from build123d import *

# Parameters (mm, degrees)
SKETCH5_R               = 2.5
BOSS_EXTRUDE2_DEPTH     = 10
CIRPATTERN2_COUNT       = 2
CUT_EXTRUDE4_REACH      = 84.468
SKETCH7_R               = 1.5
CUT_EXTRUDE5_DEPTH      = 83.46817568
SKETCH10_W              = 7.5
SKETCH10_H              = 20
BOSS_EXTRUDE3_DEPTH     = 50
CUT_EXTRUDE6_REACH      = 113.36
SKETCH11_R              = 3.75
LPATTERN1_COUNT         = 4
LPATTERN1_PITCH         = 10
MIRROR1_COPY_1_REACH    = 113.36
MIRROR1_COPY_1_SKETCH_R = 3.75
MIRROR1_COPY_2_REACH    = 113.36
MIRROR1_COPY_2_SKETCH_R = 3.75
MIRROR1_COPY_3_REACH    = 113.36
MIRROR1_COPY_3_SKETCH_R = 3.75
FILLET1_R               = 2.5


with BuildPart() as part:
    # Sketch4 → Revolve2 (revolve)
    with BuildSketch(Plane(origin=(0, 0, 0), x_dir=(0, 0, -1), z_dir=(1, 0, 0))):
        Polygon((0, 0), (50, 0), (50, -10), (53, -10), (53, 0), (56, 0), (56, 10), (53, 10), (53, 25), (50, 25), (50, 2), (0, 2), align=None)
    revolve(axis=Axis((0, 0, 0), (0, 1, 0)))

    # Sketch5 → Boss-Extrude2 (add)
    with BuildSketch(Plane(origin=(0, 2, 0), x_dir=(1, 0, 0), z_dir=(0, 1, 0))):
        with Locations(Location((-45, 0, 0), (0, 0, 270))):
            Circle(SKETCH5_R)
    boss_extrude2 = extrude(amount=BOSS_EXTRUDE2_DEPTH)

    # CirPattern2: Boss-Extrude2 ×2 about axis
    cirpattern2_axis = Axis((0.112781955, 0, 0), (0, 1, 0))
    for i in range(1, CIRPATTERN2_COUNT):
        add(boss_extrude2.rotate(cirpattern2_axis, i * 360 / CIRPATTERN2_COUNT))

    # Sketch6 → Cut-Extrude4 (cut, up to next)
    with BuildSketch(Plane(origin=(0, 2, 0), x_dir=(1, 0, 0), z_dir=(0, 1, 0)), mode=Mode.PRIVATE) as cut_extrude4_sk1:
        with BuildLine():
            Line((-5.740251485, 13.858192988), (-13.393920133, 32.335783638))
            ThreePointArc((-13.393920133, 32.335783638), (0, 35), (13.393920133, 32.335783638))
            Line((13.393920133, 32.335783638), (5.740251485, 13.858192988))
            ThreePointArc((5.740251485, 13.858192988), (0, 15), (-5.740251485, 13.858192988))
        make_face()
    cut_extrude4_tool1 = extrude(cut_extrude4_sk1.sketch, amount=-CUT_EXTRUDE4_REACH, mode=Mode.PRIVATE) & part.part
    add(cut_extrude4_tool1.solids().sort_by_distance((0, 2, -25.661711))[0], mode=Mode.SUBTRACT)

    # Sketch7 → Cut-Extrude5 (cut, through all)
    with BuildSketch(Plane(origin=(0, 2, 0), x_dir=(1, 0, 0), z_dir=(0, 1, 0))):
        with Locations(Location((0, 0, 0), (0, 0, 270))):
            Circle(SKETCH7_R)
    extrude(amount=-CUT_EXTRUDE5_DEPTH, mode=Mode.SUBTRACT)

    # Sketch10 → Boss-Extrude3 (add)
    with BuildSketch(Plane.XZ):
        with Locations((30, 0)):
            Rectangle(SKETCH10_W, SKETCH10_H)
    boss_extrude3 = extrude(amount=BOSS_EXTRUDE3_DEPTH)

    # Sketch11 → Cut-Extrude6 (cut, up to next)
    with BuildSketch(Plane.ZY.offset(-26.25), mode=Mode.PRIVATE) as cut_extrude6_sk1:
        with Locations((0, -10)):
            Circle(SKETCH11_R)
    cut_extrude6_tool1 = extrude(cut_extrude6_sk1.sketch, amount=-CUT_EXTRUDE6_REACH, mode=Mode.PRIVATE) & part.part
    cut_extrude6 = cut_extrude6_tool1.solids().sort_by_distance((26.25, -10, 0))[0]
    add(cut_extrude6, mode=Mode.SUBTRACT)

    # LPattern1: Cut-Extrude6 ×4
    with Locations(*[(0, -i * LPATTERN1_PITCH, 0) for i in range(1, LPATTERN1_COUNT)]):
        add(cut_extrude6, mode=Mode.SUBTRACT)

    # Mirror1: Boss-Extrude3, Cut-Extrude6 across plane
    add(boss_extrude3.mirror(Plane(origin=(0, 0, 0), x_dir=(0, 0, 1), z_dir=(1, 0, 0))))
    add(cut_extrude6.mirror(Plane(origin=(0, 0, 0), x_dir=(0, 0, 1), z_dir=(1, 0, 0))), mode=Mode.SUBTRACT)

    # Mirror1 copy 1 sketch → Mirror1 copy 1 (cut, up to next)
    with BuildSketch(Plane(origin=(-26.25, -10, 0), x_dir=(0, 0, 1), z_dir=(1, 0, 0)), mode=Mode.PRIVATE) as mirror1_copy_1_sk1:
        with Locations((0, 10)):
            Circle(MIRROR1_COPY_1_SKETCH_R)
    mirror1_copy_1_tool1 = extrude(mirror1_copy_1_sk1.sketch, amount=-MIRROR1_COPY_1_REACH, mode=Mode.PRIVATE) & part.part
    add(mirror1_copy_1_tool1.solids().sort_by_distance((-26.25, -20, 0))[0], mode=Mode.SUBTRACT)

    # Mirror1 copy 2 sketch → Mirror1 copy 2 (cut, up to next)
    with BuildSketch(Plane(origin=(-26.25, -20, 0), x_dir=(0, 0, 1), z_dir=(1, 0, 0)), mode=Mode.PRIVATE) as mirror1_copy_2_sk1:
        with Locations((0, 10)):
            Circle(MIRROR1_COPY_2_SKETCH_R)
    mirror1_copy_2_tool1 = extrude(mirror1_copy_2_sk1.sketch, amount=-MIRROR1_COPY_2_REACH, mode=Mode.PRIVATE) & part.part
    add(mirror1_copy_2_tool1.solids().sort_by_distance((-26.25, -30, 0))[0], mode=Mode.SUBTRACT)

    # Mirror1 copy 3 sketch → Mirror1 copy 3 (cut, up to next)
    with BuildSketch(Plane(origin=(-26.25, -30, 0), x_dir=(0, 0, 1), z_dir=(1, 0, 0)), mode=Mode.PRIVATE) as mirror1_copy_3_sk1:
        with Locations((0, 10)):
            Circle(MIRROR1_COPY_3_SKETCH_R)
    mirror1_copy_3_tool1 = extrude(mirror1_copy_3_sk1.sketch, amount=-MIRROR1_COPY_3_REACH, mode=Mode.PRIVATE) & part.part
    add(mirror1_copy_3_tool1.solids().sort_by_distance((-26.25, -40, 0))[0], mode=Mode.SUBTRACT)

    # Fillet1
    fillet1_edges = [part.edges().sort_by_distance(p)[0] for p in [
        (30, 0, -10),
        (26.25, 0, 0),
        (30, 0, 10),
        (33.75, 0, 0),
        (-30, 0, 10),
        (-33.75, 0, 0),
        (-30, 0, -10),
        (-26.25, 0, 0),
    ]]
    fillet(fillet1_edges, radius=FILLET1_R)


solid = part.part
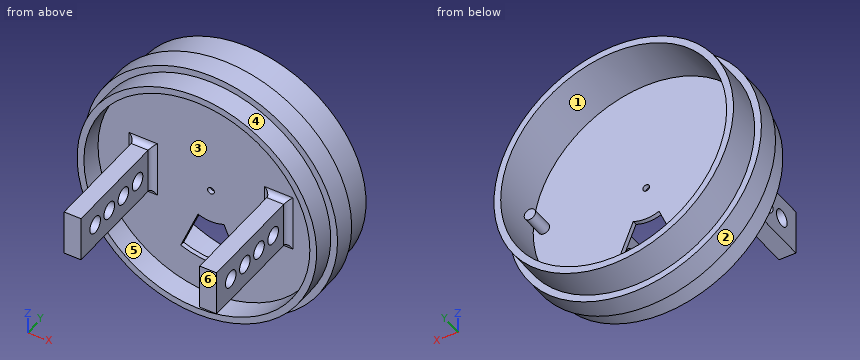
Read the model definition and answer for the solid it produces. Units are mm, in the model's axes. Face numbers are marked on the shaded views. A direction names the side the tool comes from. Round coordinates to 2 decimals unless told otherwise and drop trailing zeros. Write each loop counter-clockwise with the first axis right and the second up, starting at its lowest first coordinate (ties: lowest second). Pieces come first, ordered by that corner, then holes.
1. The part is cut by section C-C, the plane z = 0. State how many separate pieces and enclosed holes the cut face has, then the cut area to 3 significant figures.
2. The part is cut by section D-D, the plane x = -45. Determine the outline of the cut face in (y, z), then the cut area to 3 significant figures.
3. Straight lines are drawn through the part: L1, parallel to Y at x = 28, z = 0; L2, parallel to X at y = 1.4, z = 0; L3, parallel to X at y = 13, z = 0. For each, find the intervals that lie inside material, in ascending order.
4. Which of the six approach directions +Z, -Z, +X, -X, +Y, -Y give full straight-line access (tool end or side, diameter ignored) to the marked faces 1, 2 and 3?
5. The part is cut by section A-A, the plane y = -40. Determine the outline of the cut face in (x, z).
6. The part is cut by section B-B, the plane x = 0. Determine the outline of the cut face in (y, z).
7. Given pin 1 Ø4 at (x, y) = (29, -29) entering from -Z; pin 2 Ø8.5 at (y, z) = (-10, 0) entering from -X; pin 3 Ø12 at (y, z) = (-40, 0) entering from -X, each flat-ended and moving along its own axis, determine where each tip first touches the part or whether it passes through.
8. Determine the mould class of the marked faces 4, 5 and 6 for opening direction X: pulls with the +X half, pulls with the -X half, needs draft (parallel to the pull), parting line crosses it, or undercut.
Values:
1. separate pieces: 10
1. enclosed holes: 0
1. area: 869 mm2
2. outline: (-10, -28) - (0, -28) - (0, -33.33) - (10, -33.33) - (10, -28) - (25, -28) - (25, -21.79) - (2, -21.79) - (2, -2.5) - (12, -2.5) - (12, 2.5) - (2, 2.5) - (2, 21.79) - (25, 21.79) - (25, 28) - (10, 28) - (10, 33.33) - (0, 33.33) - (0, 28) - (-10, 28) - (-10, 21.79) - (0, 21.79) - (0, -21.79) - (-10, -21.79) - close
2. area: 678 mm2
3. L1: y = -50 to -43.75, -36.25 to -33.75, -26.25 to -23.75, -16.25 to -13.75, -6.25 to 2
3. L2: x = -56 to -1.5, 1.5 to 56
3. L3: x = -53 to -50, 50 to 53
4. face 1: +Y
4. face 2: +Y, -Y
4. face 3: -Y
5. outline: (-33.75, -10) - (-26.25, -10) - (-26.25, -3.75) - (-33.75, -3.75) - close; (-33.75, 3.75) - (-26.25, 3.75) - (-26.25, 10) - (-33.75, 10) - close; (26.25, -10) - (33.75, -10) - (33.75, -3.75) - (26.25, -3.75) - close; (26.25, 3.75) - (33.75, 3.75) - (33.75, 10) - (26.25, 10) - close
6. outline: (-10, -53) - (0, -53) - (0, -56) - (10, -56) - (10, -53) - (25, -53) - (25, -50) - (2, -50) - (2, -35) - (0, -35) - (0, -50) - (-10, -50) - close; (-10, 50) - (0, 50) - (0, 1.5) - (2, 1.5) - (2, 50) - (25, 50) - (25, 53) - (10, 53) - (10, 56) - (0, 56) - (0, 53) - (-10, 53) - close; (0, -15) - (2, -15) - (2, -1.5) - (0, -1.5) - close
7. pin 1: stops at z = -10
7. pin 2: stops at x = -53
7. pin 3: stops at x = -33.75
8. face 4: parting line crosses it
8. face 5: undercut
8. face 6: needs draft
